Job drawing, mm, ordinate dimensions from the low corner. One solid piece. Coordinates: 2 decimals unless noted, no trailing zeros. Loops run counter-clockwise (first coordinate to the right, second up) from the corner with the lowest first, then second, coordinate; pieces in that order, holes last. Notation, with made-up numbers: (51, 10) - (100, 10) arc R20 cw to (100, 29) - close; hole circle Ø7 at (17.25, 72.25). An arc over 180 degrees is marked (long way). Use a Markdown table: item, result. Add a question column.
1. Band-saw the part on B-B, the plane y = 1.5. Count the separate pieces of the cut face and the enclosed holes in it, plus the area to 3 significant figures.
2. Wall check: probe 1 along X at (y, z) = (0.6, 78.5); probe 2 along Z at (x, y) = (9, 2.8); probe 3 along Z at (x, y) = (7, 0.75). Give the ranges that are in metal, low to high. Write a range as [from, to].
3. Band-saw the part on D-D, the plane z = 88.5. Give the cut face in (x, y), plus the area to 3 significant figures.
4. Band-saw the part on A-A, the plane z = 125.5. Give the cut face in (x, y), plus the area to 3 significant figures.
5. Drop flat-ended pins along their axis: pin 1 (5 mm diameter, centred on x = 13.4, z = 78.5, fed in from +Y); pin 2 (10 mm diameter, centred on x = 13.4, z = 108.5, fed in from -Y). Give the stop position or say it passes through.
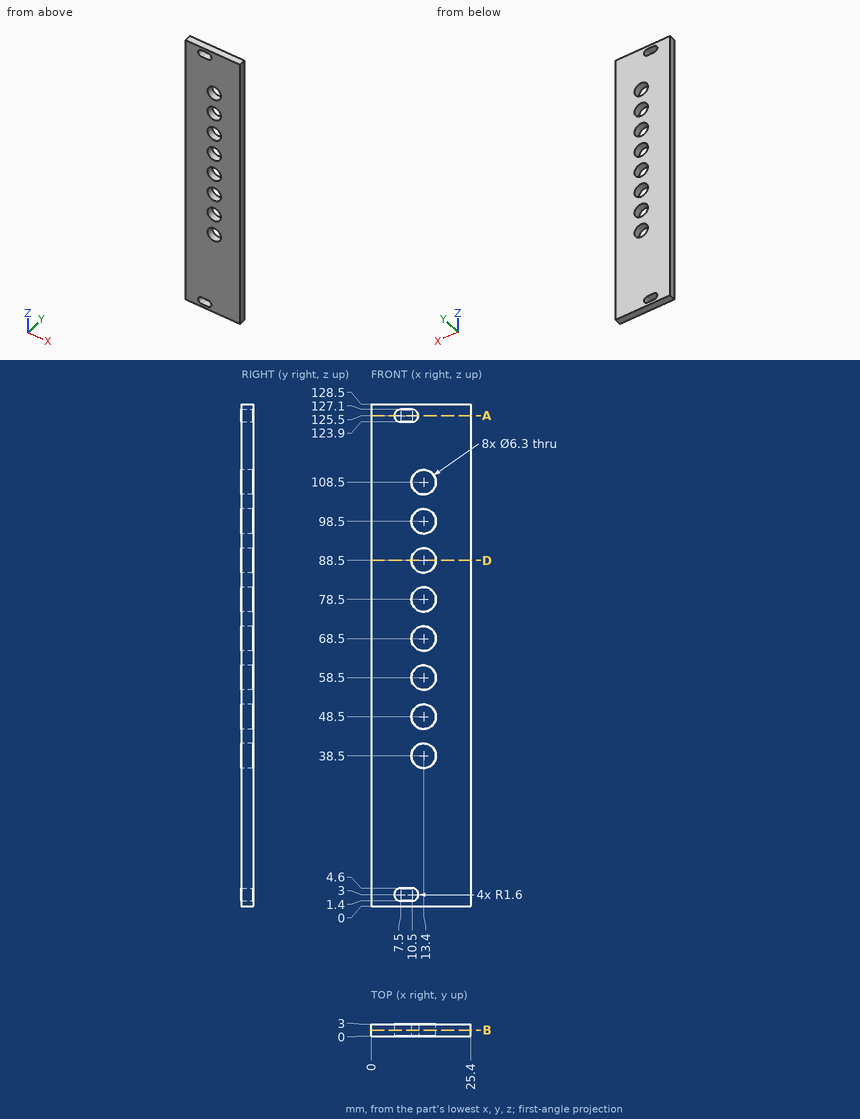
Geometry check:
| question | item | result |
|---|---|---|
| 1 | separate pieces | 1 |
| 1 | enclosed holes | 10 |
| 1 | area | 2,980 mm^2 |
| 2 | probe 1 | x = [0, 10.25], [16.55, 25.4] |
| 2 | probe 2 | z = [0, 1.4], [4.6, 123.9], [127.1, 128.5] |
| 2 | probe 3 | z = [0, 1.48], [4.52, 123.98], [127.02, 128.5] |
| 3 | outline | (0, 0) - (10.25, 0) - (10.25, 3) - (0, 3) - close; (16.55, 0) - (25.4, 0) - (25.4, 3) - (16.55, 3) - close |
| 3 | area | 57.3 mm^2 |
| 4 | outline | (0, 0) - (5.9, 0) - (5.9, 3) - (0, 3) - close; (12.1, 0) - (25.4, 0) - (25.4, 3) - (12.1, 3) - close |
| 4 | area | 57.6 mm^2 |
| 5 | pin 1 | passes through |
| 5 | pin 2 | stops at y = 0 |
